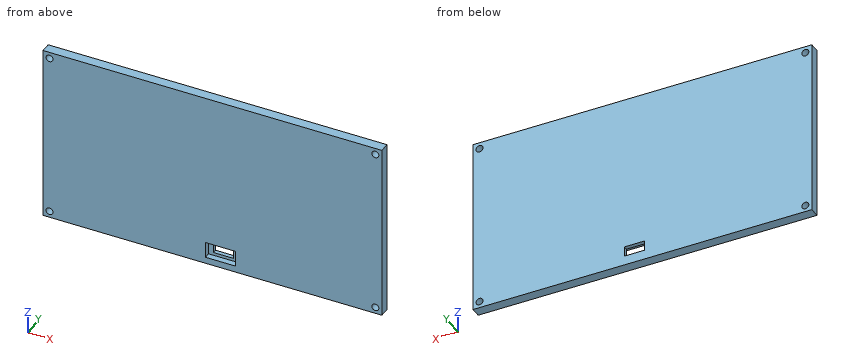
```python
from build123d import *

# Parameters (mm, degrees)
SKETCH_W        = 169.5
SKETCH_H        = 89.5
PAD_DEPTH       = 5
SKETCH001_R     = 1.75
SKETCH001_W     = 10
SKETCH001_H     = 5
POCKET_DEPTH    = 5
SKETCH002_W     = 15
SKETCH002_H     = 8
POCKET001_DEPTH = 3


with BuildPart() as part:
    # Sketch → Pad (new body)
    with BuildSketch(Plane.XZ):
        Rectangle(SKETCH_W, SKETCH_H)
    extrude(amount=PAD_DEPTH)

    # Sketch001 (on Face6 of Pad) → Pocket (cut)
    with BuildSketch(Plane.XZ.offset(5)):
        with Locations((-81.5, 41.5)):
            Circle(SKETCH001_R)
        with Locations((81.5, 41.5)):
            Circle(SKETCH001_R)
        with Locations((-81.5, -41.5)):
            Circle(SKETCH001_R)
        with Locations((81.5, -41.5)):
            Circle(SKETCH001_R)
        with Locations((4, -37.5)):
            Rectangle(SKETCH001_W, SKETCH001_H)
    extrude(amount=-POCKET_DEPTH, mode=Mode.SUBTRACT)

    # Sketch002 (on Face5 of Pocket) → Pocket001 (cut)
    with BuildSketch(Plane.XZ.offset(5)):
        with Locations((4, -37.5)):
            Rectangle(SKETCH002_W, SKETCH002_H)
    extrude(amount=-POCKET001_DEPTH, mode=Mode.SUBTRACT)


solid = part.part
```
Model file for the job. Use its own axes, mm. Give positions to 0.01 mm unless a question says otherwise; leave off trailing zeros. Write each loop counter-clockwise with the first axis right and the second up, starting at its lowest first coordinate (ties: lowest second). Pieces come first, ordered by that corner, then holes. Notation, with made-up numbers: (82, 1) -> (133, 1) arc R36 cw to (133, 39) -> close; hole circle Ø9 at (-20.75, 34). An arc over 180 degrees is marked (long way). Use CSV: the item, a comma, the result in double quotes. Start each with the question number.
1) Cut at B-B on z = 41.5. List the corners of the cut face in (x, y).
2) Drill centre line: L1, parallel to Z at x = 81.5, y = -2.55. Where is it in solid material? Low to high.
3) Pin check, flat tips, straight feed: P1, Ø2, axis at x = -4.5, z = -13.5, coming from the +Y side; P2, Ø2, axis at x = 81.5, z = 41.5, coming from the +Y side. Stop position of each tip, or through.
4) Cut at A-A on x = 81.5. List the corners of the cut face in (y, z), plus the area to 4 significant figures.
Final values:
1,outline,"(-84.75, -5) -> (-83.25, -5) -> (-83.25, 0) -> (-84.75, 0) -> close; (-79.75, -5) -> (79.75, -5) -> (79.75, 0) -> (-79.75, 0) -> close; (83.25, -5) -> (84.75, -5) -> (84.75, 0) -> (83.25, 0) -> close"
2,L1,"z = -44.75 to -43.25, -39.75 to 39.75, 43.25 to 44.75"
3,P1,"stops at y = 0"
3,P2,"passes through"
4,outline,"(-5, -44.75) -> (0, -44.75) -> (0, -43.25) -> (-5, -43.25) -> close; (-5, -39.75) -> (0, -39.75) -> (0, 39.75) -> (-5, 39.75) -> close; (-5, 43.25) -> (0, 43.25) -> (0, 44.75) -> (-5, 44.75) -> close"
4,area,"412.5 mm2"
